Model file for the job. Use its own axes, mm. Round coordinates to 2 decimals unless told otherwise and drop trailing zeros. Order: outer loops, then holes, each group sorted by start corner. A loop starts at its lowest first (then second) coordinate and runs counter-clockwise, first axis right, second up. Notation, with made-up numbers: M 49,-34.75 L 95,-34.75 A10 ccw 95,-23.75 Z; hole C 5,15.5 d8. An arc over 180 degrees is marked long. Return JSON: item names as keys, results as strings. Group by question number.
Item 1: Slice it at D-D on z = 22. Write the cut outline in (x, y).
Item 2: Pull direction Y, two halves, no side cores. Call faces 1 (the face through (7, 27.94, 0)), 2 (the face through (6.512, -14.49, 18.897)), 3 (the face through (7, 0, 27.94)): pulls with the +Y half, pulls with the -Y half, needs draft (parallel to the pull), parting line crosses it, or undercut.
Item 3: Slice it at A-A on z = 0. Write the cut outline in (x, y).
Item 4: Pin check, flat tip, straight feed: pin 1 Ø6.5 at (y, z) = (-22.55, 22.55) entering from +X. Stop position of the tip, or through.
Item 5: Probe line 1 along Y through (x, z) = (2.5, -24.5); line 2 along Z through (x, y) = (8.5, -13); line 3 along Z through (x, y) = (11.5, -8). List the from-to ranges inside material, lowest first.
Item 6: Slice it at C-C on x = 12.5. Write the cut outline in (y, z) (1 decimal).
from build123d import *

# Parameters (mm, degrees)
SKETCH1_W               = 55.88
SKETCH1_H               = 55.88
SKETCH1_R               = 23.8125
BOSS_EXTRUDE1_DEPTH     = 13.208
SKETCH5_R               = 2.54
CUT_EXTRUDE2_DEPTH      = 14.208
CUT_EXTRUDE2_DEPTH_BACK = 1


with BuildPart() as part:
    # Sketch1 → Boss-Extrude1 (new body)
    with BuildSketch(Plane(origin=(0, 0, 0), x_dir=(0, 0, -1), z_dir=(1, 0, 0))):
        Rectangle(SKETCH1_W, SKETCH1_H)
        Circle(SKETCH1_R, mode=Mode.SUBTRACT)
    extrude(amount=BOSS_EXTRUDE1_DEPTH)

    # Sketch5 → Cut-Extrude2 (cut, two sides)
    with BuildSketch(Plane(origin=(0, 0, 0), x_dir=(0, 0, -1), z_dir=(1, 0, 0))) as cut_extrude2_sk:
        with Locations((-22.551846327, -22.551846327)):
            Circle(SKETCH5_R)
        with Locations((-22.551846327, 22.551846327)):
            Circle(SKETCH5_R)
        with Locations((22.551846327, 22.551846327)):
            Circle(SKETCH5_R)
        with Locations((22.551846327, -22.551846327)):
            Circle(SKETCH5_R)
    extrude(amount=CUT_EXTRUDE2_DEPTH, mode=Mode.SUBTRACT)
    extrude(cut_extrude2_sk.sketch, amount=-CUT_EXTRUDE2_DEPTH_BACK, mode=Mode.SUBTRACT)


solid = part.part
Output values:
{
 "1": {"outline": "M 0,-27.94 L 13.21,-27.94 L 13.21,-25.03 L 0,-25.03 Z; M 0,-20.07 L 13.21,-20.07 L 13.21,-9.11 L 0,-9.11 Z; M 0,9.11 L 13.21,9.11 L 13.21,20.07 L 0,20.07 Z; M 0,25.03 L 13.21,25.03 L 13.21,27.94 L 0,27.94 Z"},
 "2": {"face 1": "pulls with the +Y half", "face 2": "undercut", "face 3": "needs draft"},
 "3": {"outline": "M 0,-27.94 L 13.21,-27.94 L 13.21,-23.81 L 0,-23.81 Z; M 0,23.81 L 13.21,23.81 L 13.21,27.94 L 0,27.94 Z"},
 "4": {"pin 1": "x = 13.21"},
 "5": {"line 1": "-27.94 to -24.18, -20.92 to 20.92, 24.18 to 27.94", "line 2": "-27.94 to -19.95, 19.95 to 27.94", "line 3": "-27.94 to -22.43, 22.43 to 27.94"},
 "6": {"outline": "M -27.9,-27.9 L 27.9,-27.9 L 27.9,27.9 L -27.9,27.9 Z; hole C -22.6,-22.6 d5.1; hole C -22.6,22.6 d5.1; hole C 0,0 d47.6; hole C 22.6,-22.6 d5.1; hole C 22.6,22.6 d5.1"}
}
